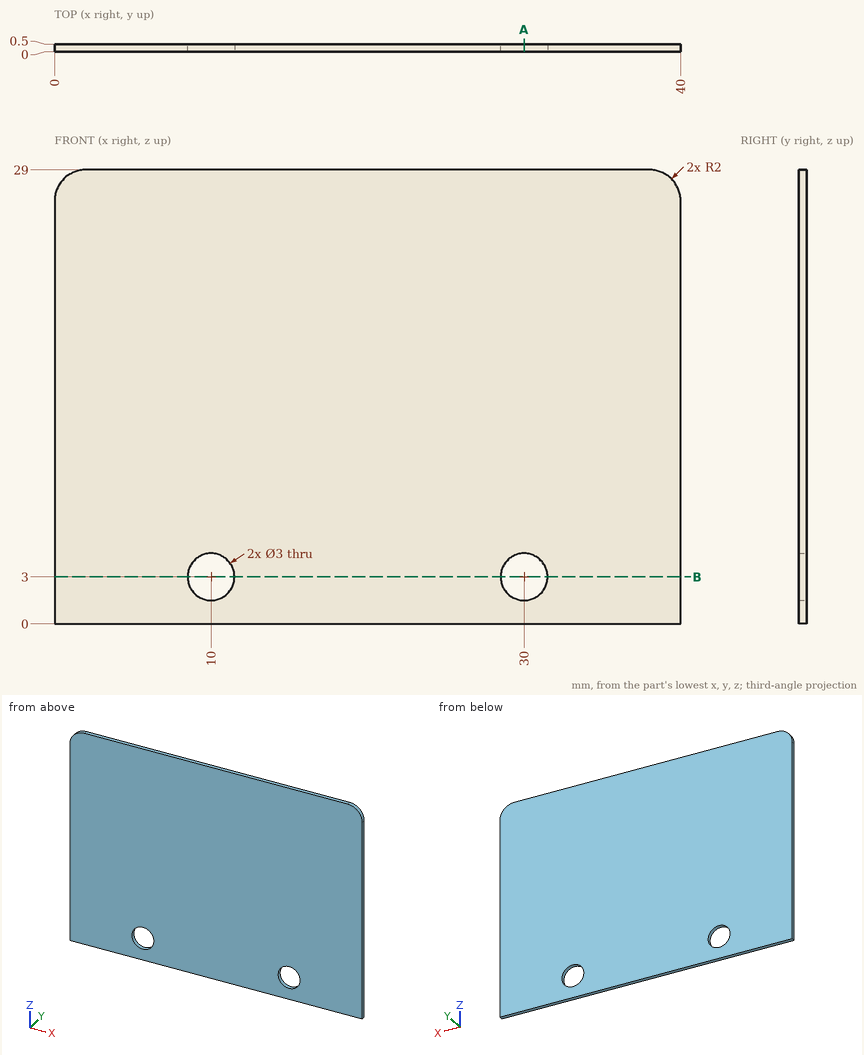
For this review, use the dimensioned drawing (mm, ordinates from the lowest corner) and the shaded views. Give positions to 0.01 mm unless a question says otherwise; leave off trailing zeros. Order: outer loops, then holes, each group sorted by start corner. A loop starts at its lowest first (then second) coordinate and runs counter-clockwise, first axis right, second up.
1) Take a section at B-B (z = 3). Give the boundary of the cut face in (x, y).
2) Insertion check: pin 1 (2.5 mm diameter, centred on x = 10, z = 3, fed in from -Y); pin 2 (3.5 mm diameter, centred on x = 30, z = 3, fed in from -Y). Each pin has a flat end and moves straight along its axis. Give the tip position at first contact, or say it passes through.
3) Wall thickness on line 1 (Z direction, x = 30, y = 0.25); line 2 (X direction, y = 0.4, z = 4.25): over which ranges is each line inside the solid? List them lowest first.
4) Take a section at A-A (x = 30). Give the boundary of the cut face in (y, z), then the cut area to 3 significant figures.
Derived:
1. outline: (0, 0) - (8.5, 0) - (8.5, 0.5) - (0, 0.5) - close; (11.5, 0) - (28.5, 0) - (28.5, 0.5) - (11.5, 0.5) - close; (31.5, 0) - (40, 0) - (40, 0.5) - (31.5, 0.5) - close
2. pin 1: passes through
2. pin 2: stops at y = 0
3. line 1: z = 0 to 1.5, 4.5 to 29
3. line 2: x = 0 to 9.17, 10.83 to 29.17, 30.83 to 40
4. outline: (0, 0) - (0.5, 0) - (0.5, 1.5) - (0, 1.5) - close; (0, 4.5) - (0.5, 4.5) - (0.5, 29) - (0, 29) - close
4. area: 13.0 mm2
